CAD build for the part. Positions are in the model's coordinates, mm. Face numbers are marked on the shaded views. A direction names the side the tool comes from. Coordinates: 2 decimals unless noted, no trailing zeros. Loops run counter-clockwise (first coordinate to the right, second up) from the corner with the lowest first, then second, coordinate; pieces in that order, holes last. Notation, with made-up numbers: (-34.5, 39.25) -> (-9.5, 39.25) arc R21 cw to (-9.5, 70.25) -> close; hole circle Ø5 at (-35, 51). An arc over 180 degrees is marked (long way). Write each question's results on one line, items separated by ' | '.
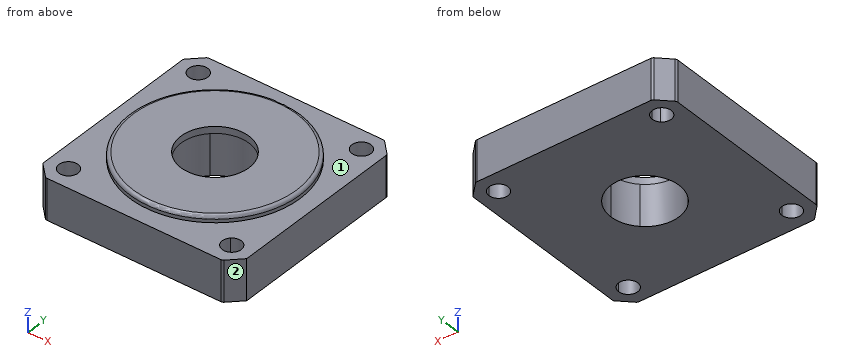
```python
from build123d import *
from build123d import SkipClean  # not in build123d's __all__

# Parameters (mm, degrees)
F1_DEPTH = 7.62
F2_R     = 15.875
F2_R_2   = 6.35
F3_DEPTH = 1.27
F4_R     = 0.635


with BuildPart() as f1:
    # F0 (on Top) → F1 (new body)
    with BuildSketch(Plane.XY):
        Polygon((16.51, 19.05), (-16.51, 19.05), (-19.05, 16.51), (-19.05, -16.51), (-16.51, -19.05), (16.51, -19.05), (19.05, -16.51), (19.05, 0), (19.05, 16.51), align=None)
        with BuildLine():
            ThreePointArc((-13.4704748936, -15.2484748936), (-16.8911327024, -15.9288860363), (-13.9912390366, -13.9912390366))
            ThreePointArc((-13.9912390366, -13.9912390366), (-13.6058170848, -14.5680637508), (-13.4704748936, -15.2484748936))
        make_face(mode=Mode.SUBTRACT)
        with BuildLine():
            ThreePointArc((17.0264748936, -15.2484748936), (14.5680637508, -16.8911327024), (13.9912390366, -13.9912390366))
            ThreePointArc((13.9912390366, -13.9912390366), (15.9288860363, -13.6058170848), (17.0264748936, -15.2484748936))
        make_face(mode=Mode.SUBTRACT)
        with BuildLine():
            ThreePointArc((-13.4704748936, 15.2484748936), (-13.6058170848, 14.5680637508), (-13.9912390366, 13.9912390366))
            ThreePointArc((-13.9912390366, 13.9912390366), (-16.8911327024, 15.9288860363), (-13.4704748936, 15.2484748936))
        make_face(mode=Mode.SUBTRACT)
        with BuildLine():
            ThreePointArc((4.4901280605, 4.4901280605), (5.8666350314, 2.4300397955), (6.35, 0))
            ThreePointArc((6.35, 0), (5.8666350314, -2.4300397955), (4.4901280605, -4.4901280605))
            ThreePointArc((4.4901280605, -4.4901280605), (0, -6.35), (-4.4901280605, -4.4901280605))
            ThreePointArc((-4.4901280605, -4.4901280605), (-6.35, 0), (-4.4901280605, 4.4901280605))
            ThreePointArc((-4.4901280605, 4.4901280605), (0, 6.35), (4.4901280605, 4.4901280605))
        make_face(mode=Mode.SUBTRACT)
        with BuildLine():
            ThreePointArc((17.0264748936, 15.2484748936), (15.9288860363, 13.6058170848), (13.9912390366, 13.9912390366))
            ThreePointArc((13.9912390366, 13.9912390366), (14.5680637508, 16.8911327024), (17.0264748936, 15.2484748936))
        make_face(mode=Mode.SUBTRACT)
    extrude(amount=F1_DEPTH)

    # F2 (on face) → F3 (join)
    with BuildSketch(Plane.XY.offset(7.62)):
        Circle(F2_R)
        Circle(F2_R_2, mode=Mode.SUBTRACT)
    with SkipClean():  # cleaning this boolean's faces spoils the solid; the shape is the same uncleaned
        extrude(amount=F3_DEPTH)

    # F4
    f4_edges = [f1.edges().sort_by_distance(p)[0] for p in [
        (-15.875, 0, 8.89),
        (-19.05, 16.51, 3.81),
        (-19.05, -16.51, 3.81),
        (-16.51, -19.05, 3.81),
        (16.51, -19.05, 3.81),
        (19.05, 16.51, 3.81),
        (16.51, 19.05, 3.81),
        (-16.51, 19.05, 3.81),
    ]]
    fillet(f4_edges, radius=F4_R)


solid = f1.part
```
Q1. Which spindle directions (+Z, -Z, +X, -X, +Y, -Y) get a long thin tool onto all of the face, cutting with end or side? Do the marked faces 1 and 2. Say none if no direction does.
Results are:
face 1: +Z | face 2: +Z, -Z, +X, -Y
Q2. Drop flat-ended pins along their axis: pin 1 (2 mm diameter, centred on x = -15.25, y = -15.25, fed in from +Z); pin 2 (4.5 mm diameter, centred on x = -15.25, y = 15.25, fed in from +Z). Give the stop position or say it passes through.
Results are:
pin 1: through | pin 2: z = 7.62
Q3. Wall check: L1, parallel to Y at x = 0, z = 7.95 (3 decimals); L2, parallel to X at y = 0, z = 7.25; L3, parallel to X at y = -14, z = 5.75. Give the ranges that are in metal, low to high. Write a range as from..to.
Results are:
L1: -15.875..-6.35, 6.35..15.875 | L2: -19.05..-6.35, 6.35..19.05 | L3: -19.05..-16.51, -13.98..13.98, 16.51..19.05
Q4. Cut at A-A on z = 6. Write the cut outline in (x, y) (3 decimals), and give its area (3 significant figures).
Results are:
outline: (-19.05, -16.247) arc R0.635 ccw to (-18.864, -16.696) -> (-16.696, -18.864) arc R0.635 ccw to (-16.247, -19.05) -> (16.247, -19.05) arc R0.635 ccw to (16.696, -18.864) -> (19.05, -16.51) -> (19.05, 16.247) arc R0.635 ccw to (18.864, 16.696) -> (16.696, 18.864) arc R0.635 ccw to (16.247, 19.05) -> (-16.247, 19.05) arc R0.635 ccw to (-16.696, 18.864) -> (-18.864, 16.696) arc R0.635 ccw to (-19.05, 16.247) -> close; hole circle Ø3.556 at (-15.248, -15.248); hole circle Ø3.556 at (-15.248, 15.248); hole circle Ø12.7 at (0, 0); hole circle Ø3.556 at (15.248, -15.248); hole circle Ø3.556 at (15.248, 15.248) | area: 1,270 mm^2
Q5. Cut at B-B on x = 0. Write the cut outline in (y, z) (3 decimals).
Results are:
outline: (-19.05, 0) -> (-6.35, 0) -> (-6.35, 8.89) -> (-15.24, 8.89) arc R0.635 ccw to (-15.875, 8.255) -> (-15.875, 7.62) -> (-19.05, 7.62) -> close; (6.35, 0) -> (19.05, 0) -> (19.05, 7.62) -> (15.875, 7.62) -> (15.875, 8.255) arc R0.635 ccw to (15.24, 8.89) -> (6.35, 8.89) -> close
